Source: three-view drawing plus pictorial views. Frame: mm from the lowest corner of the part. A direction names the side the tool comes from. Give positions to 0.01 mm unless a question says otherwise; leave off trailing zeros. Order: outer loops, then holes, each group sorted by start corner. A loop starts at its lowest first (then second) coordinate and runs counter-clockwise, first axis right, second up. Notation, with made-up numbers: (-19.75, -39.75) - (-6.75, -39.75) arc R22 cw to (-6.75, -9.75) - close; hole circle Ø7 at (-11.75, -14). An arc over 180 degrees is marked (long way). Use CSV: the item, a comma, the result in double quotes.
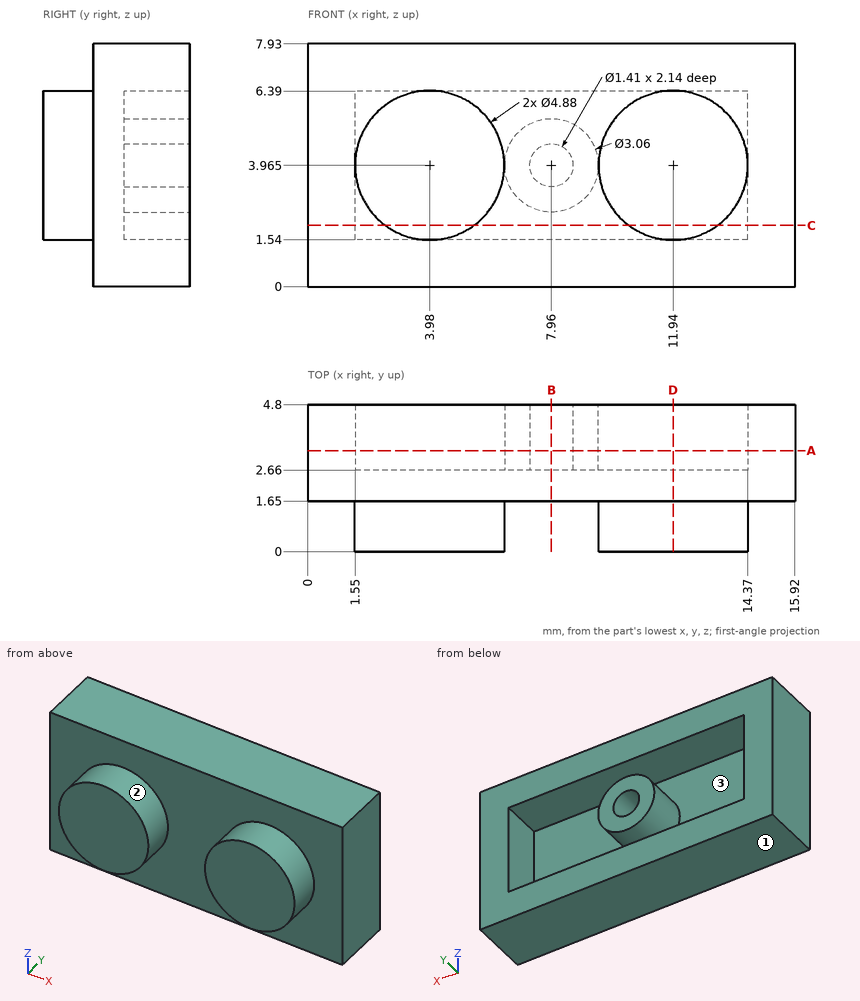
Item 1: Section C-C on z = 2. Return the cut outline in (x, y), then the cut area to 3 significant figures.
Filled in:
outline,"(0, 1.65) - (2.53, 1.65) - (2.53, 0) - (5.43, 0) - (5.43, 1.65) - (10.49, 1.65) - (10.49, 0) - (13.39, 0) - (13.39, 1.65) - (15.92, 1.65) - (15.92, 4.8) - (14.37, 4.8) - (14.37, 2.66) - (1.55, 2.66) - (1.55, 4.8) - (0, 4.8) - close"
area,"32.3 mm2"
Item 2: Material intervals for line 1 (Z direction, x = 7.96, y = 3.2) (3 decimals); line 2 (Z direction, x = 1.75, y = 2.7); line 3 (X direction, y = 4.15, z = 6.25), sorted ascending. Write a range as from..to.
Filled in:
line 1,"z = 0..1.54, 2.435..3.26, 4.67..5.495, 6.39..7.93"
line 2,"z = 0..1.54, 6.39..7.93"
line 3,"x = 0..1.55, 14.37..15.92"
Item 3: Section B-B on x = 7.96. Return the cut outline in (y, z) (3 decimals), then the cut area to 3 significant figures.
Filled in:
outline,"(1.65, 0) - (4.8, 0) - (4.8, 1.54) - (2.66, 1.54) - (2.66, 2.435) - (4.8, 2.435) - (4.8, 3.26) - (2.66, 3.26) - (2.66, 4.67) - (4.8, 4.67) - (4.8, 5.495) - (2.66, 5.495) - (2.66, 6.39) - (4.8, 6.39) - (4.8, 7.93) - (1.65, 7.93) - close"
area,"18.1 mm2"
Item 4: Set-up query: the marked faces 1, 2 and 3. Return all of +Z, -Z, +X, -X, +Y, -Y with unobstructed straight access to the full face (end or side cutting, diameter ignored); none if empty.
Filled in:
face 1,"-Z, +X, -X, +Y, -Y"
face 2,"-Y"
face 3,"+Y"
Item 5: Section A-A on y = 3.3. Return the cut outline in (x, z) (3 decimals), then the cut area to 3 significant figures.
Filled in:
outline,"(0, 0) - (15.92, 0) - (15.92, 7.93) - (0, 7.93) - close; circle Ø3.06 at (7.96, 3.965); hole (1.55, 1.54) - (14.37, 1.54) - (14.37, 6.39) - (1.55, 6.39) - close; hole circle Ø1.41 at (7.96, 3.965)"
area,"69.9 mm2"
Item 6: Section D-D on x = 11.94. Return the cut outline in (y, z) (3 decimals), then the cut area to 3 significant figures.
Filled in:
outline,"(0, 1.525) - (1.65, 1.525) - (1.65, 0) - (4.8, 0) - (4.8, 1.54) - (2.66, 1.54) - (2.66, 6.39) - (4.8, 6.39) - (4.8, 7.93) - (1.65, 7.93) - (1.65, 6.405) - (0, 6.405) - close"
area,"22.7 mm2"
